```python
from build123d import *

# Parameters (mm, degrees)
SKETCH1_W            = 55
SKETCH1_H            = 109
SKETCH1_W_2          = 45
SKETCH1_H_2          = 92
BOSS_EXTRUDE1_DEPTH  = 5
SKETCH2_R            = 1.75
CUT_EXTRUDE1_DEPTH   = 62.249489794
LPATTERN1_COUNT      = 3
LPATTERN1_PITCH      = 50
SKETCH3_W            = 7.5
SKETCH3_H            = 109
BOSS_EXTRUDE2_DEPTH  = 5
M5_CLEARANCE_HOLE1_D = 5.5
FILLET1_R            = 2


with BuildPart() as part:
    # Sketch1 → Boss-Extrude1 (new body)
    with BuildSketch(Plane.XY):
        Rectangle(SKETCH1_W, SKETCH1_H)
        Rectangle(SKETCH1_W_2, SKETCH1_H_2, mode=Mode.SUBTRACT)
    extrude(amount=BOSS_EXTRUDE1_DEPTH)

    # Sketch2 → Cut-Extrude1 (cut, through all)
    with BuildSketch(Plane.XY.offset(5)):
        with Locations((0, 50.75)):
            Circle(SKETCH2_R)
        with Locations((0, -50.75)):
            Circle(SKETCH2_R)
    extrude(amount=-CUT_EXTRUDE1_DEPTH, mode=Mode.SUBTRACT)

    # LPattern1: part ×3


with BuildPart() as part_1:
    add(part.part)
    with Locations(*[(i * LPATTERN1_PITCH, 0, 0) for i in range(1, LPATTERN1_COUNT)]):
        add(part.part)

    # Sketch3 → Boss-Extrude2 (add)
    with BuildSketch(Plane.XY.offset(5)):
        with Locations((-31.25, 0)):
            Rectangle(SKETCH3_W, SKETCH3_H)
        with Locations((131.25, 0)):
            Rectangle(SKETCH3_W, SKETCH3_H)
    extrude(amount=-BOSS_EXTRUDE2_DEPTH)

    # M5 Clearance Hole1 (through all)
    with Locations(Plane.XY.offset(5)):
        with Locations((-30, 49.5), (130, 49.5), (130, -49.5), (-30, -49.5)):
            Hole(M5_CLEARANCE_HOLE1_D / 2)

    # Fillet1
    fillet1_edges = [part_1.edges().sort_by_distance(p)[0] for p in [
        (-35, -54.5, 2.5),
        (-35, 54.5, 2.5),
        (135, 54.5, 2.5),
        (135, -54.5, 2.5),
    ]]
    fillet(fillet1_edges, radius=FILLET1_R)


solid = part_1.part
```
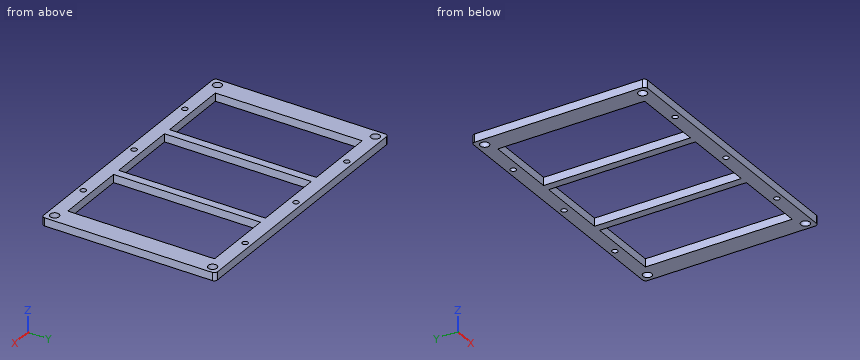
Design review of the part built by this model. Coordinates are the model's own, in mm. Coordinates: 2 decimals unless noted, no trailing zeros. Write each loop counter-clockwise with the first axis right and the second up, starting at its lowest first coordinate (ties: lowest second). Pieces come first, ordered by that corner, then holes.
1) Add section C-C (y = 41). Write out the cut boundary in (x, z).
2) Add section B-B (x = 41.5). Write out the cut boundary in (y, z).
3) Add section D-D (x = 130). Write out the cut boundary in (y, z), plus the area to 3 significant figures.
4) To check wall thickness, follow L1, parallel to Y at x = 130, z = 3.8; L2, parallel to X at y = 16, z = 1.2; L3, parallel to Y at x = 0, z = 3. State the ranges of each line that lie inside material, in increasing order.
5) Add section A-A (z = 4.15). State how many separate pieces and enclosed holes the cut face has, plus the area to 3 significant figures.
6) Insertion check: pin 1 (4 mm diameter, centred on x = 50, y = 50.75, fed in from -Z); pin 2 (3 mm diameter, centred on x = 100, y = -50.75, fed in from -Z). Each pin has a flat end and moves straight along its axis. Give the tip position at first contact, or say it passes through.
Check result:
1. outline: (-35, 0) - (-22.5, 0) - (-22.5, 5) - (-35, 5) - close; (22.5, 0) - (27.5, 0) - (27.5, 5) - (22.5, 5) - close; (72.5, 0) - (77.5, 0) - (77.5, 5) - (72.5, 5) - close; (122.5, 0) - (135, 0) - (135, 5) - (122.5, 5) - close
2. outline: (-54.5, 0) - (-46, 0) - (-46, 5) - (-54.5, 5) - close; (46, 0) - (54.5, 0) - (54.5, 5) - (46, 5) - close
3. outline: (-54.5, 0) - (-52.25, 0) - (-52.25, 5) - (-54.5, 5) - close; (-46.75, 0) - (46.75, 0) - (46.75, 5) - (-46.75, 5) - close; (52.25, 0) - (54.5, 0) - (54.5, 5) - (52.25, 5) - close
3. area: 490 mm2
4. L1: y = -54.5 to -52.25, -46.75 to 46.75, 52.25 to 54.5
4. L2: x = -35 to -22.5, 22.5 to 27.5, 72.5 to 77.5, 122.5 to 135
4. L3: y = -54.5 to -52.5, -49 to -46, 46 to 49, 52.5 to 54.5
5. separate pieces: 1
5. enclosed holes: 13
5. area: 5,950 mm2
6. pin 1: stops at z = 0
6. pin 2: passes through
